Can you work these out from the model? Positions are in its coordinate system, mm. A direction names the side the tool comes from. Round coordinates to 2 decimals unless told otherwise and drop trailing zeros. Write each loop counter-clockwise with the first axis right and the second up, starting at its lowest first coordinate (ties: lowest second). Pieces come first, ordered by that corner, then holes. Notation, with made-up numbers: M 23,9 L 52,9 A18 cw 52,33 Z; hole C 21.25,0 d11. An arc over 180 degrees is marked long. Answer as a JSON object with one key per item and string values. Group by question number.
1) Suppose I cut it at C-C, the plane z = 8.5. Write out the boundary of the cut face in (x, y) (3 decimals), and give its area (3 significant figures).
2) Suppose I cut it at B-B, the plane y = 13.5. Write out the boundary of the cut face in (x, z), and give its area (3 significant figures).
3) Please list where these lines run through material, in increasing order: L1, parallel to Z at x = 10.5, y = 27.75; L2, parallel to X at y = 4.75, z = 6; L3, parallel to Z at x = 5.5, y = 2. Write a range as [from, to].
4) I'm going to push flat-ended pins straight in: pin 1 Ø8 at (y, z) = (8, -7.5) entering from -X; pin 2 Ø8 at (y, z) = (5, -3) entering from +X. Where does each tip first touch, or does it pass through?
5) Suppose I cut it at D-D, the plane x = 5. Write out the boundary of the cut face in (y, z) (3 decimals), and give its area (3 significant figures).
6) Suppose I cut it at A-A, the plane x = 21. Write out the boundary of the cut face in (y, z) (3 decimals).
7) On a 3-axis mill with a long thin cutter (end or side, diameter ignored), from which of +Z, -Z, +X, -X, +Y, -Y can I reach the whole of each face in a straight line? I mean faces 1 (the flat face through (31.75, 14, -22)), 2 (the flat face through (4.318, 14, 0)). Say none if no direction works.
8) If we mould it in two halves opening along Z, with no side actions, what happens to faces 3 (the flat face through (16, 14, -25.4)), 4 (the flat face through (20, 14, 18.796)), 5 (the flat face through (4, 0, -4))? For each: +Z half, -Z half, draft (parallel to the pull), parting line (faces both ways), or undercut.
Solid Edge part; units mm, degrees
sketch "Sketch1" plane through (0, 0, 0) normal (0, -1, 0) x (1, 0, 0)
  line L0 (0, 25.4) -> (31.75, 25.4)
  line L1 (31.75, 25.4) -> (31.75, 18.796)
  line L2 (31.75, 18.796) -> (8.128, 18.796)
  arc A0 (8.128, 18.796) -> (4.318, 14.986) centre (8.128, 14.986) ccw
  line L3 (4.318, 14.986) -> (4.318, -14.986)
  arc A1 (4.318, -14.986) -> (8.128, -18.796) centre (8.128, -14.986) ccw
  line L4 (8.128, -18.796) -> (31.75, -18.796)
  line L5 (31.75, -18.796) -> (31.75, -25.4)
  line L6 (31.75, -25.4) -> (0, -25.4)
  line L7 (0, 25.4) -> (0, -25.4)
  dimension "D1" = 31.75
  dimension "D2" = 31.75
extrude "Protrusion1" add sketch "Sketch1" against normal blind 28.575
Results:
{
 "1": {"outline": "M 0,0 L 4.318,0 L 4.318,28.575 L 0,28.575 Z", "area": "123 mm^2"},
 "2": {"outline": "M 0,-25.4 L 31.75,-25.4 L 31.75,-18.8 L 8.13,-18.8 A3.81 cw 4.32,-14.99 L 4.32,14.99 A3.81 cw 8.13,18.8 L 31.75,18.8 L 31.75,25.4 L 0,25.4 Z", "area": "588 mm^2"},
 "3": {"L1": "[-25.4, -18.8], [18.8, 25.4]", "L2": "[0, 4.32]", "L3": "[-25.4, -17.74], [17.74, 25.4]"},
 "4": {"pin 1": "x = 0", "pin 2": "x = 4.32"},
 "5": {"outline": "M 0,-25.4 L 28.575,-25.4 L 28.575,-17.161 L 0,-17.161 Z; M 0,17.161 L 28.575,17.161 L 28.575,25.4 L 0,25.4 Z", "area": "471 mm^2"},
 "6": {"outline": "M 0,-25.4 L 28.575,-25.4 L 28.575,-18.796 L 0,-18.796 Z; M 0,18.796 L 28.575,18.796 L 28.575,25.4 L 0,25.4 Z"},
 "7": {"face 1": "+Z, -Z, +X, +Y, -Y", "face 2": "+X, +Y, -Y"},
 "8": {"face 3": "-Z half", "face 4": "undercut", "face 5": "draft"}
}
